from build123d import *

# Parameters (mm, degrees)
SKETCH1_W           = 49
SKETCH1_H           = 9
BOSS_EXTRUDE1_DEPTH = 2
SKETCH2_W           = 49
SKETCH2_H           = 3
BOSS_EXTRUDE2_DEPTH = 49
SKETCH3_R           = 1.5
SKETCH3_R_2         = 7
CUT_EXTRUDE1_DEPTH  = 3
SKETCH4_R           = 2.5
CUT_EXTRUDE2_DEPTH  = 1
SKETCH5_R           = 1.5
CUT_EXTRUDE3_DEPTH  = 2
SKETCH6_R           = 1.5
CUT_EXTRUDE4_DEPTH  = 2


with BuildPart() as part:
    # Sketch1 → Boss-Extrude1 (new body)
    with BuildSketch(Plane(origin=(0, 0, 0), x_dir=(1, 0, 0), z_dir=(0, 1, 0))):
        Rectangle(SKETCH1_W, SKETCH1_H)
    extrude(amount=BOSS_EXTRUDE1_DEPTH)

    # Sketch2 → Boss-Extrude2 (add)
    with BuildSketch(Plane(origin=(0, 2, 0), x_dir=(1, 0, 0), z_dir=(0, 1, 0))):
        with Locations((0, 3)):
            Rectangle(SKETCH2_W, SKETCH2_H)
    extrude(amount=BOSS_EXTRUDE2_DEPTH)

    # Sketch3 → Cut-Extrude1 (cut)
    with BuildSketch(Plane.XY.offset(-1.5)):
        with Locations((-9, 9.5)):
            Circle(SKETCH3_R)
        with Locations((9, 9.5)):
            Circle(SKETCH3_R)
        with Locations((-9, 42.5)):
            Circle(SKETCH3_R)
        with Locations((9, 42.5)):
            Circle(SKETCH3_R)
        with Locations((0, 18.5)):
            Circle(SKETCH3_R_2)
    extrude(amount=-CUT_EXTRUDE1_DEPTH, mode=Mode.SUBTRACT)

    # Sketch4 → Cut-Extrude2 (cut)
    with BuildSketch(Plane(origin=(0, 2, 0), x_dir=(1, 0, 0), z_dir=(0, 1, 0))):
        with Locations(Location((-21, -1.5, 0), (0, 0, 270))):
            Circle(SKETCH4_R)
        with Locations(Location((21, -1.5, 0), (0, 0, 270))):
            Circle(SKETCH4_R)
    extrude(amount=-CUT_EXTRUDE2_DEPTH, mode=Mode.SUBTRACT)

    # Sketch5 → Cut-Extrude3 (cut)
    with BuildSketch(Plane(origin=(0, 1, 0), x_dir=(1, 0, 0), z_dir=(0, 1, 0))):
        with Locations(Location((-21, -1.5, 0), (0, 0, 270))):
            Circle(SKETCH5_R)
    extrude(amount=-CUT_EXTRUDE3_DEPTH, mode=Mode.SUBTRACT)

    # Sketch6 → Cut-Extrude4 (cut)
    with BuildSketch(Plane(origin=(0, 1, 0), x_dir=(1, 0, 0), z_dir=(0, 1, 0))):
        with Locations(Location((21, -1.5, 0), (0, 0, 270))):
            Circle(SKETCH6_R)
    extrude(amount=-CUT_EXTRUDE4_DEPTH, mode=Mode.SUBTRACT)


solid = part.part
Geometry: final body of the model. Coordinates: model frame, mm. A direction names the side the tool comes from. Give positions to 0.01 mm unless a question says otherwise; leave off trailing zeros. Write each loop counter-clockwise with the first axis right and the second up, starting at its lowest first coordinate (ties: lowest second). Pieces come first, ordered by that corner, then holes. Notation, with made-up numbers: (-20.75, 11) -> (9.25, 11) arc R4 cw to (9.25, 15) -> close; hole circle Ø9 at (11, 19.5). An arc over 180 degrees is marked (long way). Answer as a JSON object with one key per item and string values.
1. Cut plane D-D on x = -21. Output: boundary loops of the cut face in (y, z).
Ans:
{"outline": "(0, -4.5) -> (51, -4.5) -> (51, -1.5) -> (2, -1.5) -> (2, -1) -> (1, -1) -> (1, 0) -> (0, 0) -> close; (0, 3) -> (1, 3) -> (1, 4) -> (2, 4) -> (2, 4.5) -> (0, 4.5) -> close"}
2. Cut plane C-C on x = -9. Output: boundary loops of the cut face in (y, z), and give its area (3 significant figures).
Ans:
{"outline": "(0, -4.5) -> (8, -4.5) -> (8, -1.5) -> (2, -1.5) -> (2, 4.5) -> (0, 4.5) -> close; (11, -4.5) -> (41, -4.5) -> (41, -1.5) -> (11, -1.5) -> close; (44, -4.5) -> (51, -4.5) -> (51, -1.5) -> (44, -1.5) -> close", "area": "147 mm^2"}
3. Cut plane A-A on y = 18.5. Output: boundary loops of the cut face in (x, z), and give its area (3 significant figures).
Ans:
{"outline": "(-24.5, -4.5) -> (-7, -4.5) -> (-7, -1.5) -> (-24.5, -1.5) -> close; (7, -4.5) -> (24.5, -4.5) -> (24.5, -1.5) -> (7, -1.5) -> close", "area": "105 mm^2"}
4. Ray query, probe 1 along X at (y, z) = (1.35, 1.5); probe 2 along Y at (x, z) = (9, -2.7); probe 3 along Y at (x, z) = (18, 0.75). Return the intervals inside material, ascending. Write a range as from..to.
Ans:
{"probe 1": "x = -24.5..-23.5, -18.5..18.5, 23.5..24.5", "probe 2": "y = 0..8, 11..41, 44..51", "probe 3": "y = 0..2"}
5. Contact query for flat-ended pins moving along their axis: pin 1 (1.5 mm diameter, centred on x = 20.5, z = 1.5, fed in from +Y); pin 2 (14.5 mm diameter, centred on x = -3.5, y = 33.5, fed in from +Z); pin 3 (4 mm diameter, centred on x = 21, z = 1.5, fed in from +Y); pin 4 (3 mm diameter, centred on x = 15.5, z = -2, fed in from -Y). Output: stop coordinate, or through.
Ans:
{"pin 1": "passes through", "pin 2": "stops at z = -1.5", "pin 3": "stops at y = 1", "pin 4": "stops at y = 0"}
6. Access query for faces 4 (the flat face through (0, 2, 1)), 5 (the flat face through (20, 1, 3)), 6 (the cylindrical face through (-9, 41, -3)). Directions: +Z, -Z, +X, -X, +Y, -Y. A direction counts if a zero-diameter tool reaches every point of the face in a straight line with its end or side. Return the directions, or none.
Ans:
{"face 4": "+Z, +X, -X, +Y", "face 5": "+Y", "face 6": "+Z, -Z"}
7. Cut plane B-B on z = -2.5. Output: boundary loops of the cut face in (x, y), and give its area (3 significant figures).
Ans:
{"outline": "(-24.5, 0) -> (24.5, 0) -> (24.5, 51) -> (-24.5, 51) -> close; hole circle Ø3 at (-9, 9.5); hole circle Ø3 at (-9, 42.5); hole circle Ø14 at (0, 18.5); hole circle Ø3 at (9, 9.5); hole circle Ø3 at (9, 42.5)", "area": "2,320 mm^2"}
8. Mould query, pull axis X, two halves, no side actions, for faces 1 (the flat face through (-24.5, 23, -3)), 2 (the cylindrical face through (-18.52, 1.51, 1.17)), 3 (the flat face through (0, 1, 4.5)). Classes: pulls with the +X half, pulls with the -X half, needs draft (parallel to the pull), parting line crosses it, or undercut.
Ans:
{"face 1": "pulls with the -X half", "face 2": "undercut", "face 3": "needs draft"}
